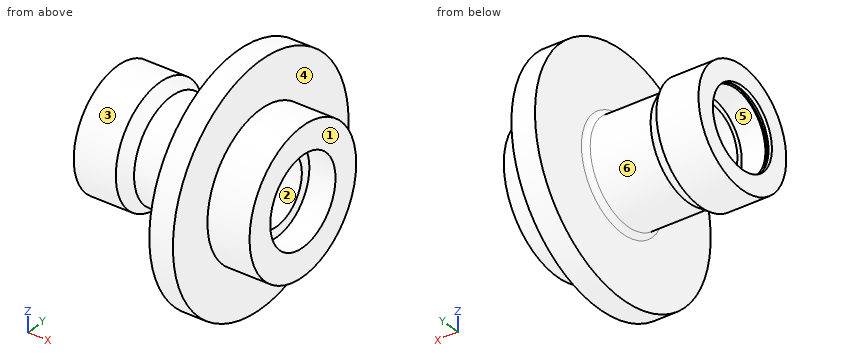
```python
from build123d import *

# Parameters (mm, degrees)
RACCORDO1_R = 3


with BuildPart() as part:
    # Schizzo1 → Rivoluzione1 (revolve)
    with BuildSketch(Plane.XY):
        Polygon((-41.225471698, 23.5), (-27.225471698, 23.5), (-27.225471698, 20), (49.424528302, 20), (49.424528302, 26), (64.924528302, 26), (64.924528302, 42.5), (39.924528302, 42.5), (39.924528302, 70), (25.924528302, 70), (25.924528302, 30), (-12.934731664, 30), (-20.075471698, 35), (-45.075471698, 35), (-45.075471698, 23.5), (-43.075471698, 23.5), (-43.075471698, 24.75), (-41.225471698, 24.75), align=None)
    revolve(axis=Axis((0, 0, 0), (1, 0, 0)))

    # Raccordo1
    raccordo1_edges = [part.edges().sort_by_distance(p)[0] for p in [
        (25.924528302, -30, 0),
    ]]
    fillet(raccordo1_edges, radius=RACCORDO1_R)


solid = part.part
```
Read the model definition and answer for the solid it produces. Units are mm, in the model's axes. Face numbers are marked on the shaded views. A direction names the side the tool comes from. Coordinates: 2 decimals unless noted, no trailing zeros. Write each loop counter-clockwise with the first axis right and the second up, starting at its lowest first coordinate (ties: lowest second). Pieces come first, ordered by that corner, then holes. Notation, with made-up numbers: (51.25, -6.75) - (58.25, -6.75) arc R19 ccw to (58.25, 1.25) - close; hole circle Ø7 at (70, 38.5). An arc over 180 degrees is marked (long way). Answer as a JSON object with one key per item and string values. Group by question number.
1. A cutting plane is placed at A-A (x = 35.5). Determine the outline of the cut face in (y, z), plus the area to 3 significant figures.
2. Which of the six approach directions +Z, -Z, +X, -X, +Y, -Y give full straight-line access (tool end or side, diameter ignored) to the marked faces 4, 5 and 6?
3. A cutting plane is placed at B-B (x = -38). Determine the outline of the cut face in (y, z).
4. A cutting plane is placed at C-C (y = -59). Determine the outline of the cut face in (x, z), plus the area to 3 significant figures.
5. The mould has two halves that part along Z. Classify the marked faces 1, 2 and 3: +Z half, -Z half, draft (parallel to the pull), parting line (faces both ways), or undercut.
6. Each of these flat-tipped pins is pushed along its axis until it touches: P1, Ø10, axis at x = 43.5, y = -8, coming from the -Z side; P2, Ø8, axis at y = 26, z = 55, coming from the +X side; P3, Ø6, axis at x = -10, z = -25.5, coming from the -Y side. Where does it stop, or does it pass through?
7. Consider L1, parallel to Z at x = -30, y = 0; L2, parallel to Z at x = -14, y = 7.5; L3, parallel to X at y = -3, z = -61.5. Determine where each line is inside the solid, lowest interval first. Write a range as [from, to].
Worked out:
{
 "1": {"outline": "circle Ø140 at (0, 0); hole circle Ø40 at (0, 0)", "area": "14,100 mm²"},
 "2": {"face 4": "+X", "face 5": "-X", "face 6": "none"},
 "3": {"outline": "circle Ø70 at (0, 0); hole circle Ø47 at (0, 0)"},
 "4": {"outline": "(25.92, -37.67) - (39.92, -37.67) - (39.92, 37.67) - (25.92, 37.67) - close", "area": "1,050 mm²"},
 "5": {"face 1": "draft", "face 2": "undercut", "face 3": "parting line"},
 "6": {"P1": "stops at z = -69.85", "P2": "stops at x = 39.92", "P3": "stops at y = -19.84"},
 "7": {"L1": "z = [-35, -23.5], [23.5, 35]", "L2": "z = [-29.82, -18.54], [18.54, 29.82]", "L3": "x = [25.92, 39.92]"}
}
